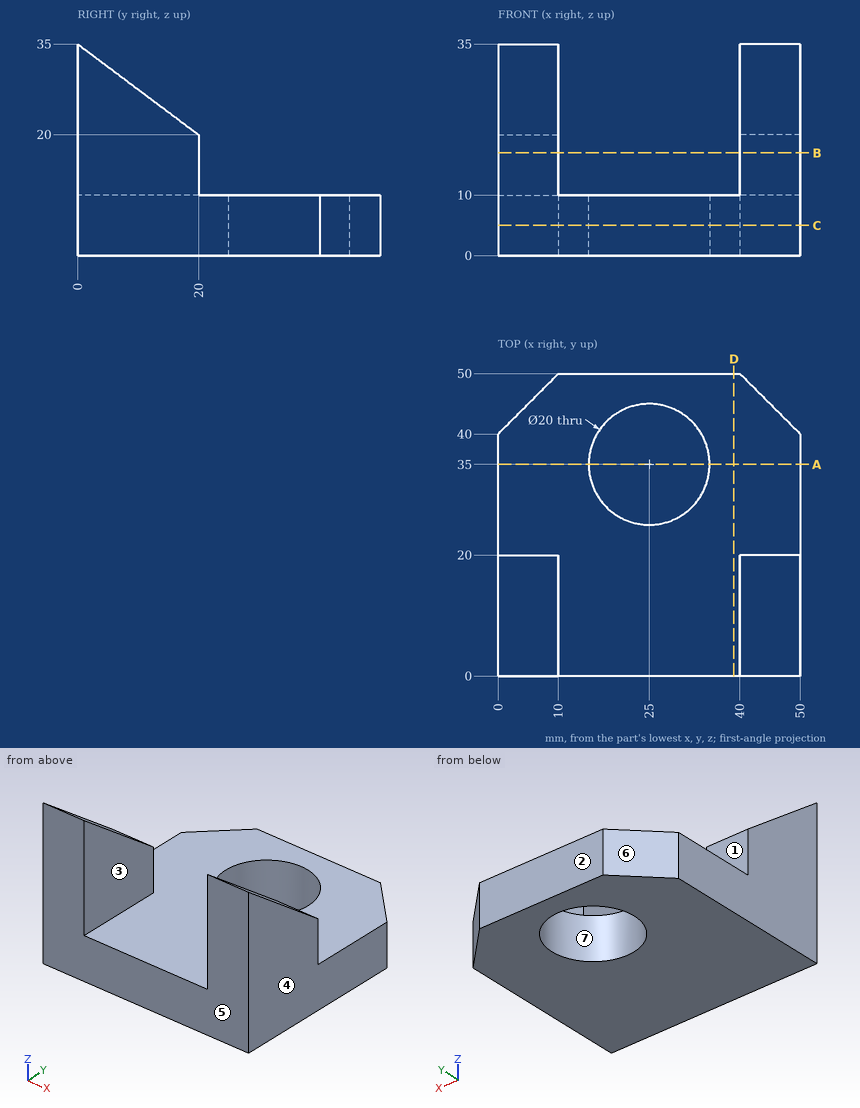
Source: three-view drawing plus pictorial views. Frame: mm from the lowest corner of the part. A direction names the side the tool comes from. Coordinates: 2 decimals unless noted, no trailing zeros. Loops run counter-clockwise (first coordinate to the right, second up) from the corner with the lowest first, then second, coordinate; pieces in that order, holes last. Notation, with made-up numbers: (40.5, 81) -> (97.5, 81) arc R32 ccw to (97.5, 107) -> close; hole circle Ø6 at (-10, 25). An arc over 180 degrees is marked (long way). Answer in a Markdown table with one row per item. Add a question column.
Q1. Section D-D on x = 39. Return the cut outline in (y, z).
Q2. Section B-B on z = 17. Return the cut outline in (x, y), and give its area (3 significant figures).
Q3. Section C-C on z = 5. Return the cut outline in (x, y).
Q4. Contact query for flat-ended pins moving along their axis: pin 1 Ø5 at (x, z) = (3, 17.5) entering from +Y; pin 2 Ø1 at (x, y) = (17.5, 8) entering from +Z. Output: stop coordinate, or through.
Q5. Ray query, line 1 along X through (y, z) = (17.5, 11); line 2 along Y through (x, z) = (25, 7.75); line 3 along Z through (x, y) = (3, 39). Return the intervals inside material, ascending.
Q6. Pull-direction query (Y, two-part tool) for the marked faces 4, 5, 6 and 7; classes: pulls with the +Y half, pulls with the -Y half, needs draft (parallel to the pull), parting line crosses it, or undercut.
Q7. Reachability of the marked faces 1, 2 and 3 from +Z, -Z, +X, -X, +Y, -Y: full face, straight path, thin tool, end or side. Return the list, or none.
Q8. Section A-A on y = 35. Return the cut outline in (x, z).
Computed values:
| question | item | result |
|---|---|---|
| 1 | outline | (0, 0) -> (50, 0) -> (50, 10) -> (0, 10) -> close |
| 2 | outline | (0, 0) -> (10, 0) -> (10, 20) -> (0, 20) -> close; (40, 0) -> (50, 0) -> (50, 20) -> (40, 20) -> close |
| 2 | area | 400 mm^2 |
| 3 | outline | (0, 0) -> (50, 0) -> (50, 40) -> (40, 50) -> (10, 50) -> (0, 40) -> close; hole circle Ø20 at (25, 35) |
| 4 | pin 1 | stops at y = 20 |
| 4 | pin 2 | stops at z = 10 |
| 5 | line 1 | x = 0 to 10, 40 to 50 |
| 5 | line 2 | y = 0 to 25, 45 to 50 |
| 5 | line 3 | z = 0 to 10 |
| 6 | face 4 | needs draft |
| 6 | face 5 | pulls with the -Y half |
| 6 | face 6 | pulls with the +Y half |
| 6 | face 7 | undercut |
| 7 | face 1 | +Z, +X, -X, +Y |
| 7 | face 2 | +Z, -Z, +X, -X, +Y |
| 7 | face 3 | +Z, +Y, -Y |
| 8 | outline | (0, 0) -> (15, 0) -> (15, 10) -> (0, 10) -> close; (35, 0) -> (50, 0) -> (50, 10) -> (35, 10) -> close |
